The figure shows three views and two pictorial views of one solid part (mm, origin at its lowest corner). Answer the questions. Coordinates: 2 decimals unless noted, no trailing zeros. Loops run counter-clockwise (first coordinate to the right, second up) from the corner with the lowest first, then second, coordinate; pieces in that order, holes last. Notation, with made-up numbers: (67.25, -18) -> (103.25, -18) arc R16 ccw to (103.25, -10) -> close; hole circle Ø5 at (81, 35.5). An arc over 180 degrees is marked (long way). Answer in a Markdown table with one row per item.
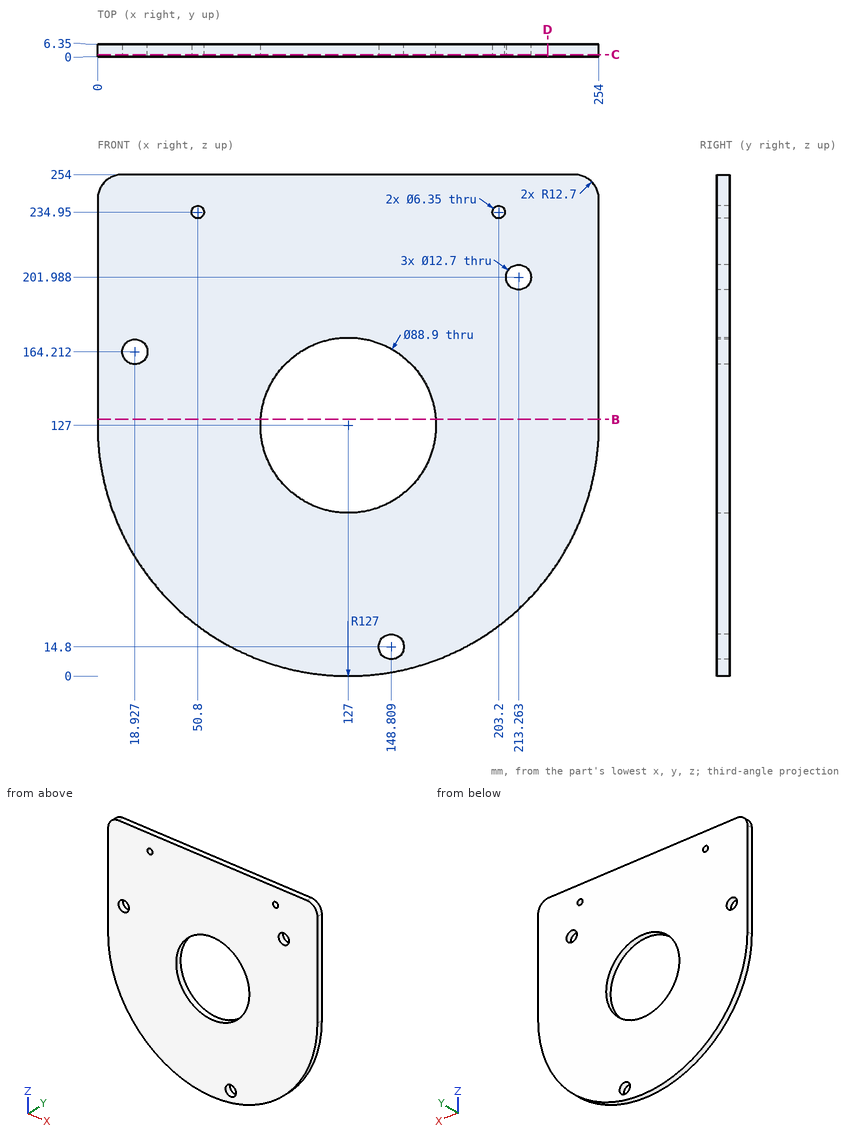
Item 1: Find the intervals of material crossed by probe 1 along X at (y, z) = (2.25, 234.95) (1 decimal); probe 2 along Z at (x, y) = (127, 4.5), in increasing order.
Findings below:
| item | result |
|---|---|
| probe 1 | x = 0 to 47.6, 54 to 200, 206.4 to 254 |
| probe 2 | z = 0 to 82.55, 171.45 to 254 |
Item 2: A cutting plane is placed at B-B, the plane z = 130. Determine the outline of the cut face in (x, y).
Findings below:
| item | result |
|---|---|
| outline | (0, 0) -> (82.65, 0) -> (82.65, 6.35) -> (0, 6.35) -> close; (171.35, 0) -> (254, 0) -> (254, 6.35) -> (171.35, 6.35) -> close |
Item 3: A cutting plane is placed at D-D, the plane x = 228. Determine the outline of the cut face in (y, z).
Findings below:
| item | result |
|---|---|
| outline | (0, 50.01) -> (6.35, 50.01) -> (6.35, 254) -> (0, 254) -> close |
Item 4: A cutting plane is placed at C-C, the plane y = 1. Count the separate pieces of the cut face and the enclosed holes in it, plus the area to 3 significant figures.
Findings below:
| item | result |
|---|---|
| separate pieces | 1 |
| enclosed holes | 6 |
| area | 50,900 mm2 |
Item 5: Flat-ended cylindrical pins translate along their axes: pin 1 Ø16.5 at (x, z) = (18.93, 164.21) entering from -Y; pin 2 Ø2 at (x, y) = (167.5, 5) entering from -Z. Find the tip coordinate at first contact, or state that the pin passes through.
Findings below:
| item | result |
|---|---|
| pin 1 | stops at y = 0 |
| pin 2 | stops at z = 6.3 |
